The listing builds one solid part. Answer for the finished solid, in the listing's coordinates (mm). A direction names the side the tool comes from. Round coordinates to 2 decimals unless told otherwise and drop trailing zeros. Order: outer loops, then holes, each group sorted by start corner. A loop starts at its lowest first (then second) coordinate and runs counter-clockwise, first axis right, second up. Notation, with made-up numbers: M -9.5,46 L -4.5,46 A19 ccw -4.5,55 Z; hole C 2,58 d1. An arc over 180 degrees is marked long. Write item = value, one per line. Start each with the question number.
(1) Which of the six approach directions +Z, -Z, +X, -X, +Y, -Y give full straight-line access (tool end or side, diameter ignored) to faces 4 (the face through (-2.461, 90.643, 29.194)), 5 (the face through (5.498, 38.821, -65.038))?
(2) Straight lines are drawn through the part: probe 1 along Z at (x, y) = (0, 92.25); probe 2 along Y at (x, z) = (-12, 55.5) (3 decimals); probe 3 along Z at (x, y) = (0, 69). For each, find the intervals that lie inside material, in ascending order. Write a range as from..to.
(3) A cutting plane is placed at C-C, the plane y = 67.5. Determine the outline of the cut face in (x, z) (1 decimal).
(4) A cutting plane is placed at D-D, the plane z = 47. Determine the outline of the cut face in (x, y) (3 decimals), and give its area (3 significant figures).
(5) A cutting plane is placed at A-A, the plane z = 20.5. Determine the outline of the cut face in (x, y) (3 decimals).
(6) Each of these flat-tipped pins is pushed along its axis until it touches: pin 1 (2 mm diameter, centred on x = -18, y = 17, fed in from +Z); pin 2 (2 mm diameter, centred on x = 5.5, y = 41.5, fed in from +Z); pin 3 (1 mm diameter, centred on x = 3.5, y = 25, fed in from +Z). Where does it stop, or does it pass through?
(7) A cutting plane is placed at B-B, the plane x = 0. Determine the outline of the cut face in (y, z) (3 decimals), and give its area (3 significant figures).
(8) For a pull along X with two mould halves and no side action, classify faces 1 (the face through (-25.364, -11, 1)), 2 (the face through (-2.461, -10.957, 29.194)), 3 (the face through (25.364, 91, -1)) as released by +X, released by -X, zero draft, split by the parting line, or undercut.
from build123d import *

# Parameters (mm, degrees)
F0_R     = 11.3530222264
F1_DEPTH = 22.225
F4_DEPTH = 79.375
F6_D     = 22.225


with BuildPart() as f1:
    # F0 (on Front) → F1 (new body)
    with BuildSketch(Plane.XZ):
        with BuildLine():
            Line((25.3637172282, -40.2771420777), (25.3637172282, 40.2771420777))
            ThreePointArc((25.3637172282, 40.2771420777), (0, 65.6408593059), (-25.3637172282, 40.2771420777))
            Line((-25.3637172282, 40.2771420777), (-25.3637172282, -40.2771420777))
            ThreePointArc((-25.3637172282, -40.2771420777), (0, -65.6408593059), (25.3637172282, -40.2771420777))
        make_face()
        with Locations((0, 40.2771420777)):
            Circle(F0_R, mode=Mode.SUBTRACT)
    extrude(amount=F1_DEPTH)


with BuildPart() as f2_1:
    # F2: copy of F1
    add(f1.part.moved(Location((0, 101.6, 0))))


with BuildPart() as f1_1:
    add(f1.part)

    add(f2_1.part)  # F4 merges F2_1
    # F3 (on face) → F4 (join, through all)
    with BuildSketch(Plane(origin=(0, 0, 0), x_dir=(-1, 0, 0), z_dir=(0, 1, 0))):
        with BuildLine():
            ThreePointArc((-25.3637172282, -40.2771420777), (0, -65.6408593059), (25.3637172282, -40.2771420777))
            ThreePointArc((25.3637172282, -40.2771420777), (0, -14.9134248495), (-25.3637172282, -40.2771420777))
        make_face()
    extrude(amount=F4_DEPTH)

    # F6 (through all)
    with Locations(Plane(origin=(0, 101.6, 0), x_dir=(-1, 0, 0), z_dir=(0, 1, 0))):
        with Locations((0, -40.2771420777)):
            Hole(F6_D / 2)


solid = f1_1.part
Reported:
q1.face_4 = +Y, -Y
q1.face_5 = none
q2.probe_1 = -65.64..-51.39, -29.16..28.92, 51.63..65.64
q2.probe_2 = -22.225..0, 79.375..101.6
q2.probe_3 = -65.64..-51.39, -29.16..-14.91
q3.outline = C 0,-40.3 d50.7; hole C 0,-40.3 d22.2
q4.outline = M -24.457,-22.225 L -9.148,-22.225 L -9.148,0 L -24.457,0 Z; M -24.457,79.375 L -9.148,79.375 L -9.148,101.6 L -24.457,101.6 Z; M 9.148,-22.225 L 24.457,-22.225 L 24.457,0 L 9.148,0 Z; M 9.148,79.375 L 24.457,79.375 L 24.457,101.6 L 9.148,101.6 Z
q4.area = 1,360 mm²
q5.outline = M -25.364,-22.225 L 25.364,-22.225 L 25.364,0 L -25.364,0 Z; M -25.364,79.375 L 25.364,79.375 L 25.364,101.6 L -25.364,101.6 Z
q6.pin_1 = -21.45
q6.pin_2 = -15.32
q6.pin_3 = -15.09
q7.outline = M -22.225,-65.641 L 101.6,-65.641 L 101.6,-51.39 L -22.225,-51.39 Z; M -22.225,-29.165 L 101.6,-29.165 L 101.6,28.924 L 79.375,28.924 L 79.375,-14.913 L 0,-14.913 L 0,28.924 L -22.225,28.924 Z; M -22.225,51.63 L 0,51.63 L 0,65.641 L -22.225,65.641 Z; M 79.375,51.63 L 101.6,51.63 L 101.6,65.641 L 79.375,65.641 Z
q7.area = 6,100 mm²
q8.face_1 = released by -X
q8.face_2 = undercut
q8.face_3 = released by +X
